Geometry check sheet. Reference: the model listing, model coordinates, mm. Face numbers are marked on the shaded views. A direction names the side the tool comes from. Round coordinates to 2 decimals unless told otherwise and drop trailing zeros. Write each loop counter-clockwise with the first axis right and the second up, starting at its lowest first coordinate (ties: lowest second). Pieces come first, ordered by that corner, then holes.
Item 1: Scan lines: probe 1 along X at (y, z) = (5.25, -10); probe 2 along X at (y, z) = (0.75, -15); probe 3 along X at (y, z) = (-1.75, -26). Record each from-to range of solid material in increasing order.
Item 2: Cross-section at C-C (z = -21). Enter the section's corners in (x, y), then the cut area to 3 significant figures.
Item 3: Access from +Z, -Z, +X, -X, +Y, -Y to the whole of each face (thin tool, end or side, straight path). Record for the marked faces 1 and 2.
Item 4: Cross-section at A-A (z = 1.5). Enter the section's corners in (x, y), then the cut area to 3 significant figures.
Item 5: Cross-section at B-B (y = 3). Enter the section's corners in (x, z).
Item 6: Depth check by flat-ended pin: P1, Ø0.6, axis at y = 1, z = -36.5, coming from the -X side; P2, Ø1, axis at y = 0.5, z = 36, coming from the +X side; P3, Ø0.6, axis at y = 0.5, z = 1, coming from the -X side. Enter the tip coordinate at first touch or a pass-through.
Item 7: Cross-section at D-D (x = -8). Enter the section's corners in (y, z).
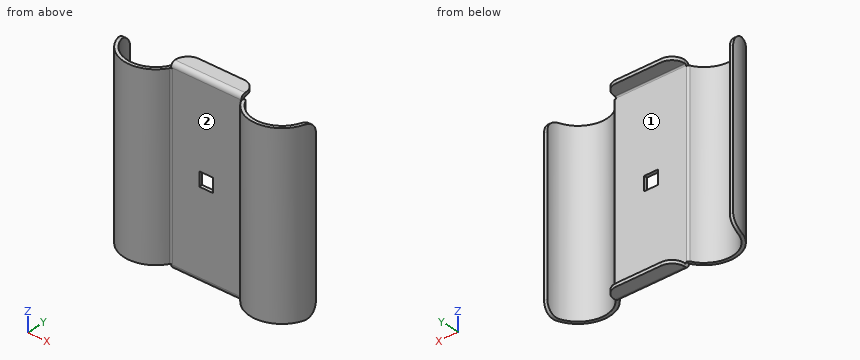
from build123d import *

# Parameters (mm, degrees)
SKETCH1_W                      = 28
SKETCH1_H                      = 74
BOSS_EXTRUDE1_DEPTH            = 1.3
EDGE_FLANGE1_STRIP_W           = 6.2
EDGE_FLANGE1_STRIP_H           = 1.3
EDGE_FLANGE1_STRIP_CUT_DEPTH   = 28
EDGE_FLANGE1_STRIP_2_W         = 6.2
EDGE_FLANGE1_STRIP_2_H         = 1.3
EDGE_FLANGE1_STRIP_CUT_2_DEPTH = 28
EDGE_FLANGE1_DEPTH             = 28
EDGE_FLANGE1_BEND_DEPTH        = 28
FILLET1_R                      = 5
SKETCH16_W                     = 5.5
SKETCH16_H                     = 5.5
CUT_EXTRUDE1_DEPTH             = 41.174618853
BOSS_EXTRUDE2_DEPTH            = 35
FILLET2_R                      = 5
FILLET3_R                      = 1


# Sheet-metal steps are written as plain solids
with BuildPart() as part:
    # Sketch1 → Boss-Extrude1 (new body)
    with BuildSketch(Plane(origin=(0, 0, 0), x_dir=(1, 0, 0), z_dir=(0, 1, 0))):
        Rectangle(SKETCH1_W, SKETCH1_H)
    extrude(amount=BOSS_EXTRUDE1_DEPTH)

    # Edge-Flange1 strip (across the edge) → Edge-Flange1 strip cut (cut)
    with BuildSketch(Plane(origin=(14, 1.3, -37), x_dir=(0, 0, 1), z_dir=(-1, 0, 0))):
        with Locations((-1.3, -0.65)):
            Rectangle(EDGE_FLANGE1_STRIP_W, EDGE_FLANGE1_STRIP_H)
    extrude(amount=EDGE_FLANGE1_STRIP_CUT_DEPTH, mode=Mode.SUBTRACT)

    # Edge-Flange1 strip 2 (across the edge) → Edge-Flange1 strip cut 2 (cut)
    with BuildSketch(Plane(origin=(-14, 1.3, 37), x_dir=(0, 0, -1), z_dir=(1, 0, 0))):
        with Locations((-1.3, -0.65)):
            Rectangle(EDGE_FLANGE1_STRIP_2_W, EDGE_FLANGE1_STRIP_2_H)
    extrude(amount=EDGE_FLANGE1_STRIP_CUT_2_DEPTH, mode=Mode.SUBTRACT)

    # Edge-Flange1 section (across the edge) → Edge-Flange1 (add)
    with BuildSketch(Plane(origin=(14, 1.3, -37), x_dir=(0, 0, 1), z_dir=(-1, 0, 0))):
        with BuildLine():
            Line((0, 0.5), (0, 5.7))
            Line((0, 5.7), (1.3, 5.7))
            Line((1.3, 5.7), (1.3, 0.5))
            ThreePointArc((1.3, 0.5), (1.446446609, 0.146446609), (1.8, 0))
            Line((1.8, 0), (1.8, -1.3))
            ThreePointArc((1.8, -1.3), (0.527207794, -0.772792206), (0, 0.5))
        make_face()
    extrude(amount=EDGE_FLANGE1_DEPTH)

    # Edge-Flange1 section 2 (across the edge) → Edge-Flange1 bend (add)
    with BuildSketch(Plane(origin=(-14, 1.3, 37), x_dir=(0, 0, -1), z_dir=(1, 0, 0))):
        with BuildLine():
            Line((0, 0.5), (0, 5.7))
            Line((0, 5.7), (1.3, 5.7))
            Line((1.3, 5.7), (1.3, 0.5))
            ThreePointArc((1.3, 0.5), (1.446446609, 0.146446609), (1.8, 0))
            Line((1.8, 0), (1.8, -1.3))
            ThreePointArc((1.8, -1.3), (0.527207794, -0.772792206), (0, 0.5))
        make_face()
    extrude(amount=EDGE_FLANGE1_BEND_DEPTH)

    # Fillet1
    fillet1_edges = [part.edges().sort_by_distance(p)[0] for p in [
        (14, 7, -36.35),
        (-14, 7, -36.35),
        (-14, 7, 36.35),
        (14, 7, 36.35),
    ]]
    fillet(fillet1_edges, radius=FILLET1_R)

    # Sketch16 → Cut-Extrude1 (cut, through all)
    with BuildSketch(Plane.XZ):
        Rectangle(SKETCH16_W, SKETCH16_H)
    extrude(amount=-CUT_EXTRUDE1_DEPTH, mode=Mode.SUBTRACT)

    # Sketch17 → Boss-Extrude2 (add, symmetric)
    with BuildSketch(Plane.XY):
        with BuildLine():
            Line((-36.411176225, 7), (-37.716721927, 7))
            ThreePointArc((-37.716721927, 7), (-28.02937954, -6.381761823), (-13.403830412, 1.3))
            Line((-13.403830412, 1.3), (-14.812491114, 1.3))
            ThreePointArc((-14.812491114, 1.3), (-28.03717688, -5.040214789), (-36.411176225, 7))
        make_face()
    boss_extrude2 = extrude(amount=BOSS_EXTRUDE2_DEPTH, both=True)

    # Mirror1: Boss-Extrude2 across plane
    add(boss_extrude2.mirror(Plane(origin=(0, 0, 0), x_dir=(0, 0, 1), z_dir=(1, 0, 0))))

    # Fillet2
    fillet2_edges = [part.edges().sort_by_distance(p)[0] for p in [
        (-37.063949076, 7, -35),
        (-37.063949076, 7, 35),
        (37.063949076, 7, 35),
        (37.063949076, 7, -35),
    ]]
    fillet(fillet2_edges, radius=FILLET2_R)

    # Fillet3
    fillet3_edges = [part.edges().sort_by_distance(p)[0] for p in [
        (-14, 0, 0),
        (-14.812491114, 1.3, 0),
        (14, 0, 0),
        (14.812491114, 1.3, 0),
    ]]
    fillet(fillet3_edges, radius=FILLET3_R)


solid = part.part
Resolved:
1. probe 1: x = -37.75 to -36.45, 36.45 to 37.75
1. probe 2: x = -36.67 to -35.22, -15.08 to 15.08, 35.22 to 36.67
1. probe 3: x = -35.18 to -33.49, -16.81 to -15.12, 15.12 to 16.81, 33.49 to 35.18
2. outline: (-37.72, 7) arc R12.61 ccw to (-14.28, -0.49) arc R1 cw to (-13.41, 0) - (13.41, 0) arc R1 cw to (14.28, -0.49) arc R12.61 ccw to (37.72, 7) - (36.41, 7) arc R11.31 cw to (15.07, 0.75) arc R1 ccw to (14.18, 1.3) - (-14.18, 1.3) arc R1 ccw to (-15.07, 0.75) arc R11.31 cw to (-36.41, 7) - close
2. area: 124 mm2
3. face 1: +Y
3. face 2: +Z, -Z, -Y
4. outline: (-37.72, 7) arc R12.61 ccw to (-14.28, -0.49) arc R1 cw to (-13.41, 0) - (-2.75, 0) - (-2.75, 1.3) - (-14.18, 1.3) arc R1 ccw to (-15.07, 0.75) arc R11.31 cw to (-36.41, 7) - close; (2.75, 0) - (13.41, 0) arc R1 cw to (14.28, -0.49) arc R12.61 ccw to (37.72, 7) - (36.41, 7) arc R11.31 cw to (15.07, 0.75) arc R1 ccw to (14.18, 1.3) - (2.75, 1.3) - close
4. area: 117 mm2
5. outline: (-37.43, -34.9) - (-36.09, -34.9) - (-36.09, 34.9) - (-37.43, 34.9) - close; (-13.9, -37) - (13.9, -37) - (13.9, -35.7) - (-13.9, -35.7) - close; (-13.9, 35.7) - (13.9, 35.7) - (13.9, 37) - (-13.9, 37) - close; (36.09, -34.9) - (37.43, -34.9) - (37.43, 34.9) - (36.09, 34.9) - close
6. P1: stops at x = -14
6. P2: stops at x = 14
6. P3: stops at x = -36.69
7. outline: (0, -35.2) arc R1.8 ccw to (1.8, -37) - (7, -37) - (7, -35.7) - (1.8, -35.7) arc R0.5 cw to (1.3, -35.2) - (1.3, 35.2) arc R0.5 cw to (1.8, 35.7) - (7, 35.7) - (7, 37) - (1.8, 37) arc R1.8 ccw to (0, 35.2) - close
